Answer from the drawing. Dimensions are ordinates in mm from the lowest x, y and z of the part. Give positions to 0.01 mm unless a question says otherwise; leave off trailing zeros. Loops run counter-clockwise (first coordinate to the right, second up) from the corner with the lowest first, then second, coordinate; pieces in that order, holes last. Notation, with made-up numbers: (10.5, -22.5) - (31.5, -22.5) arc R17 ccw to (31.5, 5.5) - close; hole circle Ø4 at (61.5, 75.25). An arc over 180 degrees is marked (long way). One line per item, written item: value.
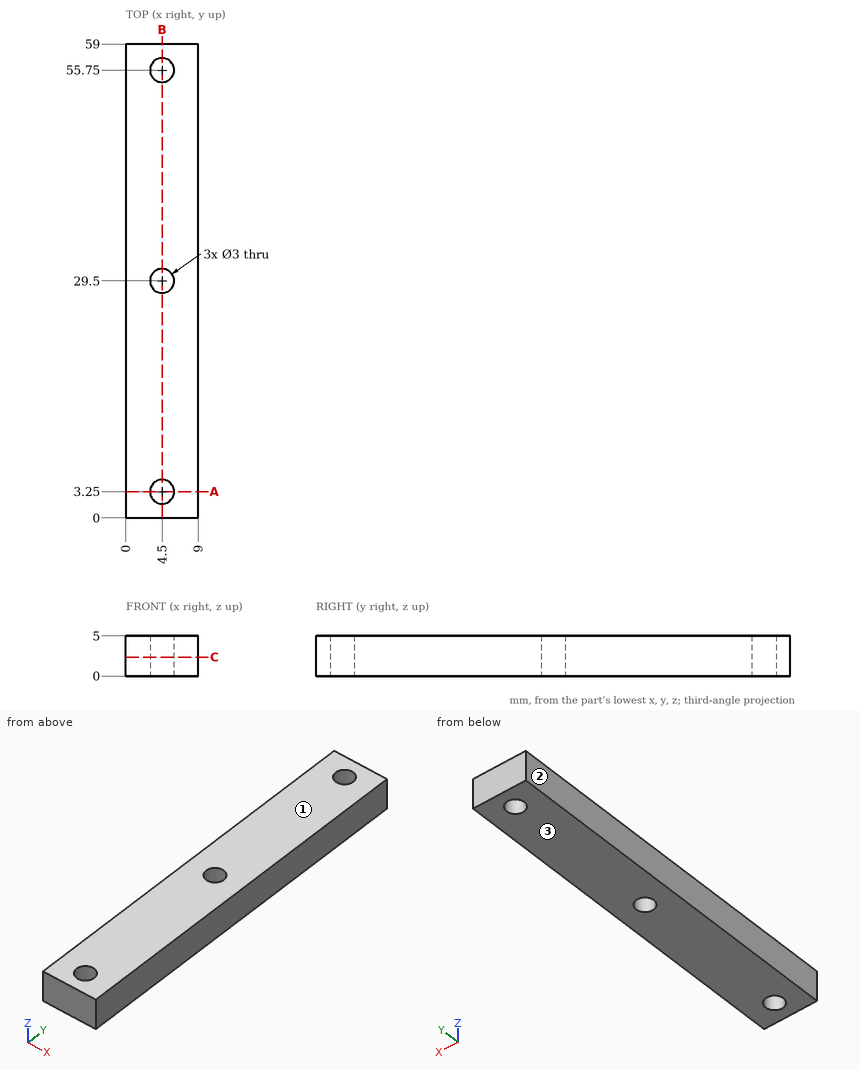
1. Section B-B (x = 4.5) is taken. Write down the section's boundary in (y, z).
Output:
outline: (0, 0) - (1.75, 0) - (1.75, 5) - (0, 5) - close; (4.75, 0) - (28, 0) - (28, 5) - (4.75, 5) - close; (31, 0) - (54.25, 0) - (54.25, 5) - (31, 5) - close; (57.25, 0) - (59, 0) - (59, 5) - (57.25, 5) - close
2. Find the intervals of material crossed by line 1 along Y through (x, z) = (4.5, 2.6); line 2 along Y through (x, z) = (5, 0.85), in increasing order.
Output:
line 1: y = 0 to 1.75, 4.75 to 28, 31 to 54.25, 57.25 to 59
line 2: y = 0 to 1.84, 4.66 to 28.09, 30.91 to 54.34, 57.16 to 59
3. The mould has two halves that part along Z. Classify the marked faces 1, 2 and 3: released by +Z, released by -Z, zero draft, split by the parting line, or undercut.
Output:
face 1: released by +Z
face 2: zero draft
face 3: released by -Z
4. Section C-C (z = 2.35) is taken. Write down the section's boundary in (x, y), and give its area (3 significant figures).
Output:
outline: (0, 0) - (9, 0) - (9, 59) - (0, 59) - close; hole circle Ø3 at (4.5, 3.25); hole circle Ø3 at (4.5, 29.5); hole circle Ø3 at (4.5, 55.75)
area: 510 mm²
5. Flat-ended cylindrical pins translate along their axes: pin 1 Ø4 at (x, y) = (1.5, 8.5) entering from -Z; pin 2 Ø1.8 at (x, y) = (4.5, 29.5) entering from +Z. Find the tip coordinate at first contact, or state that the pin passes through.
Output:
pin 1: stops at z = 0
pin 2: passes through
6. Section A-A (y = 3.25) is taken. Write down the section's boundary in (x, z).
Output:
outline: (0, 0) - (3, 0) - (3, 5) - (0, 5) - close; (6, 0) - (9, 0) - (9, 5) - (6, 5) - close
